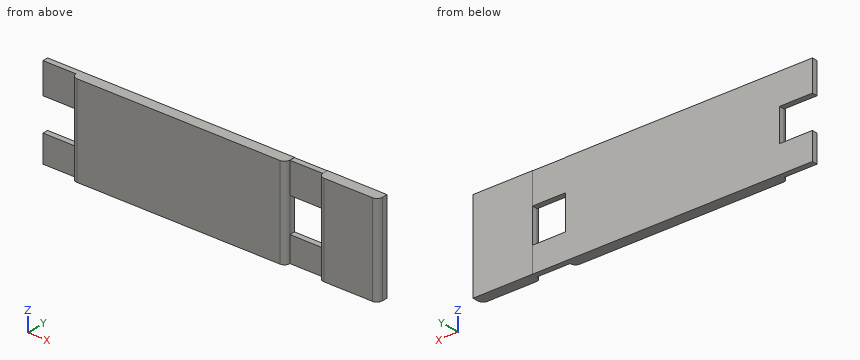
from build123d import *

# Parameters (mm, degrees)
BOSS_EXTRUDE4_DEPTH   = 50
BOSS_EXTRUDE4_2_DEPTH = 50
SKETCH7_W             = 17
SKETCH7_H             = 3
SKETCH7_W_2           = 14
BOSS_EXTRUDE5_DEPTH   = 18
SKETCH8_W             = 17
SKETCH8_H             = 3
SKETCH8_W_2           = 15
BOSS_EXTRUDE6_DEPTH   = 18


with BuildPart() as part:
    # Sketch6 → Boss-Extrude4 (new body)
    with BuildSketch(Plane.XY.offset(-2000)):
        with BuildLine():
            Line((24.966787002, 344.25912611), (24.966787002, 347.264784988))
            Line((24.966787002, 347.264784988), (-7.533155287, 347.203538294))
            Line((-7.533155287, 347.203538294), (-7.527501746, 344.203543621))
            ThreePointArc((-7.527501746, 344.203543621), (-6.644825993, 342.083882928), (-4.521853532, 341.209202489))
            Line((-4.521853532, 341.209202489), (21.972440543, 341.259131437))
            ThreePointArc((21.972440543, 341.259131437), (24.090105234, 342.139805537), (24.966787002, 344.25912611))
        make_face()
    extrude(amount=BOSS_EXTRUDE4_DEPTH)



with BuildPart() as body_2:
    # Sketch6 → Boss-Extrude4 2 (new body)
    with BuildSketch(Plane.XY.offset(-2000)):
        with BuildLine():
            Line((-25.527469784, 344.169622375), (-25.533123325, 347.169617048))
            Line((-25.533123325, 347.169617048), (-142.327839016, 346.949515419))
            Line((-142.327839016, 346.949515419), (-142.322185475, 343.949520746))
            ThreePointArc((-142.322185475, 343.949520746), (-141.439509722, 341.829860053), (-139.316537261, 340.955179614))
            Line((-139.316537261, 340.955179614), (-28.521810916, 341.163974161))
            ThreePointArc((-28.521810916, 341.163974161), (-26.402150223, 342.046649914), (-25.527469784, 344.169622375))
        make_face()
    extrude(amount=BOSS_EXTRUDE4_2_DEPTH)


with BuildPart() as part_1:
    add(part.part)

    add(body_2.part)  # Boss-Extrude5 merges body 2
    # Sketch7 → Boss-Extrude5 (add)
    with BuildSketch(Plane(origin=(-6.878819882, -0.012963253, 0), x_dir=(0, 0, 1), z_dir=(-0.9999982243025385, -0.001884513669318331, 0))):
        with Locations((-1958.612984199, 345.717118099)):
            Rectangle(SKETCH7_W, SKETCH7_H)
        with Locations((-1993, 345.717118099)):
            Rectangle(SKETCH7_W_2, SKETCH7_H)
    extrude(amount=BOSS_EXTRUDE5_DEPTH)

    # Sketch8 → Boss-Extrude6 (add)
    with BuildSketch(Plane(origin=(-141.673503611, -0.266986128, 0), x_dir=(0, 0, 1), z_dir=(-0.9999982243025385, -0.001884513669318331, 0))):
        with Locations((-1958.5, 345.717118099)):
            Rectangle(SKETCH8_W, SKETCH8_H)
        with Locations((-1992.5, 345.717118099)):
            Rectangle(SKETCH8_W_2, SKETCH8_H)
    extrude(amount=BOSS_EXTRUDE6_DEPTH)


solid = part_1.part
Read the model definition and answer for the solid it produces. Units are mm, in the model's axes. Give positions to 0.01 mm unless a question says otherwise; leave off trailing zeros. Write each loop counter-clockwise with the first axis right and the second up, starting at its lowest first coordinate (ties: lowest second). Pieces come first, ordered by that corner, then holes. Notation, with made-up numbers: (-38, 60.25) -> (-26, 60.25) arc R13 ccw to (-26, 77.25) -> close; hole circle Ø10 at (-17.75, -22.5). An arc over 180 degrees is marked (long way). Answer as a JSON object with one key per item and string values. Group by question number.
1) Consider L1, parallel to X at y = 345.5, z = -1983; L2, parallel to X at y = 344, z = -1965; L3, parallel to Y at x = 13.5, z = -1960. Determine where each line is inside the solid, lowest interval first. Write a range as from..to.
2) Find section B-B (z = -1953). Write down the section's boundary in (x, y), and give its area (3 significant figures).
3) Find section C-C (y = 342.75). Write down the section's boundary in (x, z), and give its area (3 significant figures).
4) Find section A-A (z = -1969). Write down the section's boundary in (x, y), and give its area (3 significant figures).
5) Find section D-D (x = -12.5). Write down the section's boundary in (y, z), and give its area (3 significant figures).
6) Each of these flat-tipped pins is pushed along its axis until it touches: P1, Ø2.5, axis at x = -20, y = 346, coming from the +Z side; P2, Ø1, axis at x = -119.5, z = -1981, coming from the +Y side; P3, Ø8, axis at x = -41, z = -1956, coming from the +Y side. Where does it stop, or does it pass through?
Values follow:
{
 "1": {"L1": "x = -142.33..-25.53, -7.53..24.97", "L2": "x = -160.32..-25.53, -7.52..24.96", "L3": "y = 341.24..347.24"},
 "2": {"outline": "(-160.33, 346.92) -> (-160.32, 343.92) -> (-142.32, 343.95) arc R3 ccw to (-139.32, 340.96) -> (-28.52, 341.16) arc R3 ccw to (-25.53, 344.17) -> (-7.53, 344.2) arc R3 ccw to (-4.52, 341.21) -> (21.97, 341.26) arc R3 ccw to (24.97, 344.26) -> (24.97, 347.26) -> close", "area": "996 mm2"},
 "3": {"outline": "(-142.07, -2000) -> (-25.88, -2000) -> (-25.88, -1950) -> (-142.07, -1950) -> close; (-7.15, -2000) -> (24.56, -2000) -> (24.56, -1950) -> (-7.15, -1950) -> close", "area": "7,390 mm2"},
 "4": {"outline": "(-142.33, 346.95) -> (-142.32, 343.95) arc R3 ccw to (-139.32, 340.96) -> (-28.52, 341.16) arc R3 ccw to (-25.53, 344.17) -> (-25.53, 347.17) -> close; (-7.53, 344.2) arc R3 ccw to (-4.52, 341.21) -> (21.97, 341.26) arc R3 ccw to (24.97, 344.26) -> (24.97, 347.26) -> (-7.53, 347.2) -> close", "area": "888 mm2"},
 "5": {"outline": "(344.19, -2000) -> (347.19, -2000) -> (347.19, -1986) -> (344.19, -1986) -> close; (344.19, -1967.11) -> (347.19, -1967.11) -> (347.19, -1950.11) -> (344.19, -1950.11) -> close", "area": "93.0 mm2"},
 "6": {"P1": "stops at z = -1950.11", "P2": "stops at y = 346.99", "P3": "stops at y = 347.15"}
}
